Work out the finished part from the listing and answer in its coordinate system (mm). Face numbers are marked on the shaded views. A direction names the side the tool comes from. Round coordinates to 2 decimals unless told otherwise and drop trailing zeros. Write each loop counter-clockwise with the first axis right and the second up, starting at its lowest first coordinate (ties: lowest second). Pieces come first, ordered by that corner, then holes. Notation, with made-up numbers: (52, 35.25) -> (62, 35.25) arc R27 ccw to (62, 62.25) -> close; hole circle Ø1 at (-15.75, 83). An arc over 180 degrees is marked (long way). One line per item, written item: value.
```python
from build123d import *

# Parameters (mm, degrees)
SM_BASE_FLANGE_1_DEPTH = 12.5
HOLE_WIZARD_M4_1_D     = 4.5


# Sheet-metal steps are written as plain solids
with BuildPart() as part:
    # Sketch 1 → 基体-法兰1 (new, symmetric)
    with BuildSketch(Plane(origin=(0, 0, 0), x_dir=(1, 0, 0), z_dir=(0, 1, 0))):
        with BuildLine():
            Line((0, 0), (0, -28))
            ThreePointArc((0, -28), (0.292893219, -28.707106781), (1, -29))
            Line((1, -29), (7.8, -29))
            ThreePointArc((7.8, -29), (9.567766953, -29.732233047), (10.3, -31.5))
            Line((10.3, -31.5), (10.3, -49))
            Line((10.3, -49), (8.8, -49))
            Line((8.8, -49), (8.8, -31.5))
            ThreePointArc((8.8, -31.5), (8.507106781, -30.792893219), (7.8, -30.5))
            Line((7.8, -30.5), (1, -30.5))
            ThreePointArc((1, -30.5), (-0.767766953, -29.767766953), (-1.5, -28))
            Line((-1.5, -28), (-1.5, 0))
            Line((-1.5, 0), (0, 0))
        make_face()
    extrude(amount=SM_BASE_FLANGE_1_DEPTH, both=True)

    # M4 间隙孔1 (through all)
    with Locations(Plane.ZY.offset(-8.8)):
        with Locations((44, 7.5), (44, -7.5)):
            Hole(HOLE_WIZARD_M4_1_D / 2)


solid = part.part
```
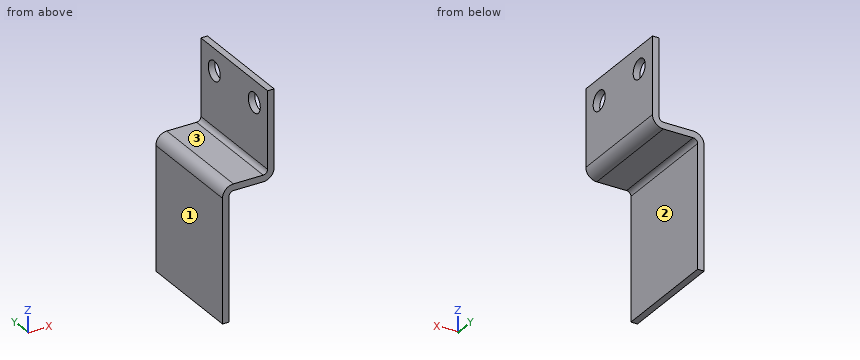
(1) A tool of negligible diameter and unlimited length cuts with its end or side. For the marked faces 1, 2 and 3, from which of +Z, -Z, +X, -X, +Y, -Y can it reach the whole face along a straight path? Write none if from no direction.
Reported:
face 1: +Z, -Z, -X, +Y, -Y
face 2: -Z, +X, +Y, -Y
face 3: +Z, -X, +Y, -Y
(2) Find section D-D on x = 6.25. Give the vertices of the cut face in (y, z).
Reported:
outline: (-12.5, 29) -> (12.5, 29) -> (12.5, 30.5) -> (-12.5, 30.5) -> close
(3) Consider probe 1 along Y at (x, z) = (9.55, 44); probe 2 along X at (y, z) = (-3.75, 44); probe 3 along Z at (x, y) = (1.5, -4.75). Determine where each line is inside the solid, lowest interval first.
Reported:
probe 1: y = -12.5 to -9.75, -5.25 to 5.25, 9.75 to 12.5
probe 2: x = 8.8 to 10.3
probe 3: z = 29 to 30.5
(4) Find section A-A on y = 7.5. Give the vertices of the cut face in (x, z).
Reported:
outline: (-1.5, 0) -> (0, 0) -> (0, 28) arc R1 cw to (1, 29) -> (7.8, 29) arc R2.5 ccw to (10.3, 31.5) -> (10.3, 41.75) -> (8.8, 41.75) -> (8.8, 31.5) arc R1 cw to (7.8, 30.5) -> (1, 30.5) arc R2.5 ccw to (-1.5, 28) -> close; (8.8, 46.25) -> (10.3, 46.25) -> (10.3, 49) -> (8.8, 49) -> close
(5) Flat-ended cylindrical pins translate along their axes: pin 1 Ø2 at (x, y) = (4.5, 4.5) entering from +Z; pin 2 Ø4 at (x, y) = (5.5, 5.5) entering from -Z; pin 3 Ø8 at (y, z) = (6.5, 36.5) entering from -X. Find the tip coordinate at first contact, or state that the pin passes through.
Reported:
pin 1: stops at z = 30.5
pin 2: stops at z = 29
pin 3: stops at x = 8.8
(6) Find section C-C on y = 4. Give the vertices of the cut face in (x, z), plus the area to 3 significant figures.
Reported:
outline: (-1.5, 0) -> (0, 0) -> (0, 28) arc R1 cw to (1, 29) -> (7.8, 29) arc R2.5 ccw to (10.3, 31.5) -> (10.3, 49) -> (8.8, 49) -> (8.8, 31.5) arc R1 cw to (7.8, 30.5) -> (1, 30.5) arc R2.5 ccw to (-1.5, 28) -> close
area: 86.7 mm2
(7) Find section B-B on z = 44. Give the vertices of the cut face in (x, y), plus the area to 3 significant figures.
Reported:
outline: (8.8, -12.5) -> (10.3, -12.5) -> (10.3, -9.75) -> (8.8, -9.75) -> close; (8.8, -5.25) -> (10.3, -5.25) -> (10.3, 5.25) -> (8.8, 5.25) -> close; (8.8, 9.75) -> (10.3, 9.75) -> (10.3, 12.5) -> (8.8, 12.5) -> close
area: 24.0 mm2
